from build123d import *

# Parameters (mm, degrees)
SKETCH1_W           = 50
SKETCH1_H           = 100
BOSS_EXTRUDE1_DEPTH = 6
SKETCH2_R           = 1.5
CUT_EXTRUDE1_DEPTH  = 112.964280018
FILLET2_R           = 1.5
CHAMFER1_SIZE2      = 16.484864517
CHAMFER1_SIZE       = 6
FILLET3_R           = 10


with BuildPart() as part:
    # Sketch1 → Boss-Extrude1 (new body)
    with BuildSketch(Plane(origin=(0, 0, 0), x_dir=(1, 0, 0), z_dir=(0, 1, 0))):
        with Locations((25, -50)):
            Rectangle(SKETCH1_W, SKETCH1_H)
    extrude(amount=BOSS_EXTRUDE1_DEPTH)

    # Sketch2 → Cut-Extrude1 (cut, through all)
    with BuildSketch(Plane(origin=(50, 0, 0), x_dir=(0, 0, -1), z_dir=(1, 0, 0))):
        with Locations((-5, 3)):
            Circle(SKETCH2_R)
    extrude(amount=-CUT_EXTRUDE1_DEPTH, mode=Mode.SUBTRACT)

    # Fillet2
    fillet2_edges = [part.edges().sort_by_distance(p)[0] for p in [
        (25, 6, 0),
        (25, 0, 0),
    ]]
    fillet(fillet2_edges, radius=FILLET2_R)

    # Chamfer1
    chamfer1_edges = [part.edges().sort_by_distance(p)[0] for p in [
        (25, 6, 100),
    ]]
    chamfer1_side = [part.faces().sort_by_distance(p)[0] for p in [
        (25, 5.88, 100),
    ]]
    chamfer(chamfer1_edges, length=CHAMFER1_SIZE - 0.0001, length2=CHAMFER1_SIZE2 - 0.0001, reference=chamfer1_side[0])  # a hair under: the kernel refuses the full size

    # Fillet3
    fillet3_edges = [part.edges().sort_by_distance(p)[0] for p in [
        (25, 6, 83.515235483),
    ]]
    fillet(fillet3_edges, radius=FILLET3_R)


solid = part.part
Build history of the part. All positions in model axes, mm. Round coordinates to 2 decimals unless told otherwise and drop trailing zeros. Order: outer loops, then holes, each group sorted by start corner. A loop starts at its lowest first (then second) coordinate and runs counter-clockwise, first axis right, second up. Notation, with made-up numbers: M 76,12 L 116,12 A30 ccw 116,46 Z; hole C -19,-26 d4. An arc over 180 degrees is marked long. Use CSV: the item, a comma, the result in double quotes. Start each with the question number.
(1) Mould opens along Y. For faces 1 (the face through (25.4, 2.1, 6.2)), 2 (the face through (25.35, 5.844, 83.513)), 3 (the face through (25, 3, 0)) say: +Y half, -Y half, draft (parallel to the pull), parting line (faces both ways), or undercut.
(2) Drill centre lines: probe 1 along Y at (x, z) = (17, 5); probe 2 along Y at (x, z) = (40.5, 92); probe 3 along Y at (x, z) = (28, 90). Where is each one in solid material? Low to high.
(3) Cut at A-A on z = 5. List the corners of the cut face in (x, y).
(4) Cut at C-C on y = 3. List the corners of the cut face in (x, z).
(5) Flat gauge pin, fed straight in: P1, Ø1.5, axis at x = 9.5, y = 0.5, coming from the -Z side. Where does the tip first touch, or does it go through?
Findings:
1,face 1,"undercut"
1,face 2,"+Y half"
1,face 3,"draft"
2,probe 1,"y = 0 to 1.5, 4.5 to 6"
2,probe 2,"y = 0 to 2.91"
2,probe 3,"y = 0 to 3.64"
3,outline,"M 0,0 L 50,0 L 50,1.5 L 0,1.5 Z; M 0,4.5 L 50,4.5 L 50,6 L 0,6 Z"
4,outline,"M 0,0 L 50,0 L 50,3.5 L 0,3.5 Z; M 0,6.5 L 50,6.5 L 50,91.76 L 0,91.76 Z"
5,P1,"stops at z = 0.02"
